from build123d import *

# Parameters (mm, degrees)
F0_W     = 65
F0_H     = 45
F1_DEPTH = 50
F2_R     = 10
F3_T     = -5
F4_W     = 50
F4_H     = 1.5
F5_DEPTH = 5
F6_R     = 1
F7_F1_R  = 0.7499
F7_F2_R  = 0.75
F8_R     = 2


# Not quite as in the source:
# - a fillet or chamfer is up to 0.001 mm smaller than in the source, because OpenCascade refuses the exact size


with BuildPart() as f1:
    # F0 (on Top) → F1 (new body)
    with BuildSketch(Plane.XY):
        Rectangle(F0_W, F0_H)
    extrude(amount=F1_DEPTH)

    # F2
    f2_edges = [f1.edges().sort_by_distance(p)[0] for p in [
        (32.5, -22.5, 25),
        (-32.5, -22.5, 25),
        (-32.5, 22.5, 25),
        (32.5, 22.5, 25),
    ]]
    fillet(f2_edges, radius=F2_R)

    # F3 (hollow: no face is removed)
    offset(amount=F3_T, mode=Mode.SUBTRACT)

    # F4 (on face) → F5 (cut, through all)
    with BuildSketch(Plane(origin=(0, 0, 0), x_dir=(1, 0, 0), z_dir=(0, 0, -1))):
        with Locations((0, -2.25)):
            Rectangle(F4_W, F4_H)
    extrude(amount=-F5_DEPTH, mode=Mode.SUBTRACT)

    # F6
    f6_edges = [f1.edges().sort_by_distance(p)[0] for p in [
        (0, -22.5, 0),
        (32.5, 0, 50),
        (29.571068, -19.571068, 50),
        (29.571068, 19.571068, 50),
        (0, -22.5, 50),
        (0, 22.5, 50),
        (-29.571068, -19.571068, 50),
        (-29.571068, 19.571068, 50),
        (-32.5, 0, 50),
        (32.5, 0, 0),
        (29.571068, -19.571068, 0),
        (29.571068, 19.571068, 0),
        (0, 22.5, 0),
        (-29.571068, -19.571068, 0),
        (-29.571068, 19.571068, 0),
        (-32.5, 0, 0),
    ]]
    fillet(f6_edges, radius=F6_R)

    # F7: fillet of radius 0.75 on 6 edges, made by hand

    # F7_f1 (radius 0.75 in the source; OpenCascade refuses exactly that, so slightly less here)
    f7_f1_edges = [f1.edges().sort_by_distance(p)[0] for p in [
        (-25, 1.5, 2.5),
        (-25, 3, 2.5),
        (25, 3, 2.5),
        (25, 1.5, 2.5),
    ]]
    fillet(f7_f1_edges, radius=F7_F1_R)

    # F7_f2
    f7_f2_edges = [f1.edges().sort_by_distance(p)[0] for p in [
        (0, 1.5, 0),
        (0, 3, 0),
        (-24.7803593752, 2.7803593752, 0),
        (24.7803593752, 2.7803593752, 0),
        (24.7803593752, 1.7196406248, 0),
        (-24.7803593752, 1.7196406248, 0),
    ]]
    fillet(f7_f2_edges, radius=F7_F2_R)

    # F8
    f8_edges = [f1.edges().sort_by_distance(p)[0] for p in [
        (27.5, 0, 5),
        (0, 17.5, 45),
        (26.035534, 16.035534, 5),
        (26.035534, -16.035534, 5),
        (0, 17.5, 5),
        (0, -17.5, 5),
        (-26.035534, 16.035534, 5),
        (-26.035534, -16.035534, 5),
        (-27.5, 0, 5),
        (27.5, 0, 45),
        (26.035534, 16.035534, 45),
        (26.035534, -16.035534, 45),
        (0, -17.5, 45),
        (-26.035534, 16.035534, 45),
        (-26.035534, -16.035534, 45),
        (-27.5, 0, 45),
    ]]
    fillet(f8_edges, radius=F8_R)


solid = f1.part
Check sheet for the modelled part. Datum: model origin and axes. Units: mm. A direction names the side the tool comes from. Give positions to 0.01 mm unless a question says otherwise; leave off trailing zeros. Loops run counter-clockwise (first coordinate to the right, second up) from the corner with the lowest first, then second, coordinate; pieces in that order, holes last. Notation, with made-up numbers: M 15.25,42.5 L 56.25,42.5 A19 cw 56.25,62.5 Z; hole C 76,66 d1. An arc over 180 degrees is marked long. Return JSON: item names as keys, results as strings. Group by question number.
1. Cross-section at C-C on z = 46. Record the boundary of the cut face in (x, y), plus the area to 3 significant figures.
2. Cross-section at D-D on x = 14. Record the boundary of the cut face in (y, z).
3. Tool access check on faces 1 (the flat face through (0, 17.5, 25)), 2 (the flat face through (32.5, 0, 25)), 3 (the flat face through (0, 1.5, 3)). Record the directions out of +Z, -Z, +X, -X, +Y, -Y that give a thin tool (end or side, any length) a straight path to the whole face; none if there is none.
4. Cross-section at A-A on y = -11. Record the boundary of the cut face in (x, z), plus the area to 3 significant figures.
5. Go/stop test with flat-tipped pins: pin 1 (4 mm diameter, centred on y = 15, z = 28.5, fed in from +X); pin 2 (5 mm diameter, centred on x = 24.5, z = 5.5, fed in from +Y). Record where each tip stops, or that it passes through.
6. Mould release check, pull along Z, two halves, no side actions. Record for faces 4 (the cylindrical face through (-26.93, 0.17, 44.4)), 5 (the cylindrical face through (26.93, -0.18, 44.4)), 6 (the flat face through (-32.5, 0, 25)), 7 (the flat face through (0, 0, 50)): released by +Z, released by -Z, zero draft, split by the parting line, or undercut.
7. Thickness scan on L1, parallel to X at y = -3, z = 11; L2, parallel to Z at x = 6, y = 6.5; L3, parallel to Y at x = -17.5, z = 21. Record the ranges inside material, lowest first.
Return value:
{
 "1": {"outline": "M -32.5,-12.5 A10 ccw -22.5,-22.5 L 22.5,-22.5 A10 ccw 32.5,-12.5 L 32.5,12.5 A10 ccw 22.5,22.5 L -22.5,22.5 A10 ccw -32.5,12.5 Z", "area": "2,840 mm^2"},
 "2": {"outline": "M -22.5,1 A1 ccw -21.5,0 L 0.75,0 A0.75 ccw 1.5,0.75 L 1.5,5 L -15.5,5 A2 cw -17.5,7 L -17.5,43 A2 cw -15.5,45 L 15.5,45 A2 cw 17.5,43 L 17.5,7 A2 cw 15.5,5 L 3,5 L 3,0.75 A0.75 ccw 3.75,0 L 21.5,0 A1 ccw 22.5,1 L 22.5,49 A1 ccw 21.5,50 L -21.5,50 A1 ccw -22.5,49 Z"},
 "3": {"face 1": "none", "face 2": "+Z, -Z, +X, +Y, -Y", "face 3": "-Z"},
 "4": {"outline": "M -32.5,1 A1 ccw -31.5,0 L 31.5,0 A1 ccw 32.5,1 L 32.5,49 A1 ccw 31.5,50 L -31.5,50 A1 ccw -32.5,49 Z; hole M -27.5,7 A2 ccw -25.5,5 L 25.5,5 A2 ccw 27.5,7 L 27.5,43 A2 ccw 25.5,45 L -25.5,45 A2 ccw -27.5,43 Z", "area": "1,050 mm^2"},
 "5": {"pin 1": "x = 32.49", "pin 2": "y = 22.5"},
 "6": {"face 4": "undercut", "face 5": "undercut", "face 6": "zero draft", "face 7": "released by +Z"},
 "7": {"L1": "-32.5 to -27.5, 27.5 to 32.5", "L2": "0 to 5, 45 to 50", "L3": "-22.5 to -17.5, 17.5 to 22.5"}
}
